Work out the finished part from the listing and answer in its coordinate system (mm). Face numbers are marked on the shaded views. A direction names the side the tool comes from. Coordinates: 2 decimals unless noted, no trailing zeros. Loops run counter-clockwise (first coordinate to the right, second up) from the corner with the lowest first, then second, coordinate; pieces in that order, holes last. Notation, with made-up numbers: (65.5, 50) -> (91.5, 50) arc R31 cw to (91.5, 74) -> close; hole circle Ø8 at (-34.75, -30). An arc over 180 degrees is marked (long way). One line per question, with ' | ' between items.
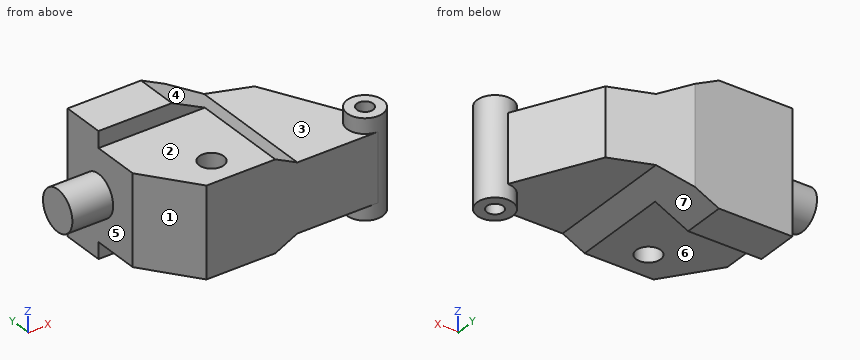
```python
from build123d import *

# Parameters (mm, degrees)
EXTRUDE_1_DEPTH          = 75
SKETCH_2_W               = 185.8
SKETCH_2_H               = 57.3
CUT_EXTRUDE_2_DEPTH      = 120
CUT_EXTRUDE_3_DEPTH      = 400
SKETCH_5_R               = 21.9
EXTRUDE_2_DEPTH          = 60
SKETCH_6_R               = 10
CUT_EXTRUDE_4_DEPTH      = 200
SKETCH_8_R               = 15
CUT_EXTRUDE_5_DEPTH      = 21
CUT_EXTRUDE_5_DEPTH_BACK = 131
SKETCH_9_R               = 25
EXTRUDE_3_DEPTH          = 50


with BuildPart() as part:
    # 草图1 → 凸台-拉伸1 (new body, symmetric)
    with BuildSketch(Plane.XY):
        Polygon((-119.6, 172.501416068), (0, 172.501416068), (86.979350222, 141.023763122), (136.480359145, 43.8), (136.480359145, 0), (-73.719640855, 0), (-119.6, 61.701416068), align=None)
    extrude(amount=EXTRUDE_1_DEPTH, both=True)

    # 草图2 → 切除-拉伸2 (cut)
    with BuildSketch(Plane(origin=(0, 0, 0), x_dir=(1, 0, 0), z_dir=(0, 1, 0))):
        with Locations((-51.7, 83.65)):
            Rectangle(SKETCH_2_W, SKETCH_2_H)
        with Locations((-51.7, -83.65)):
            Rectangle(SKETCH_2_W, SKETCH_2_H)
    extrude(amount=CUT_EXTRUDE_2_DEPTH, mode=Mode.SUBTRACT)

    # 草图3 → 切除-拉伸3 (cut)
    with BuildSketch(Plane(origin=(0, 172.501416068, 0), x_dir=(1, 0, 0), z_dir=(0, 1, 0))):
        Polygon((-64.837283081, 92.42032951), (245.362716919, 92.42032951), (245.362716919, 41.62032951), (37.776604868, 41.62032951), align=None)
        Polygon((37.776604868, -41.62032951), (-64.837283081, -92.42032951), (245.362716919, -92.42032951), (245.362716919, -41.62032951), align=None)
    extrude(amount=-CUT_EXTRUDE_3_DEPTH, mode=Mode.SUBTRACT)

    # 草图5 → 凸台-拉伸2 (add, symmetric)
    with BuildSketch(Plane.XY):
        with Locations((136.480359145, 21.9)):
            Circle(SKETCH_5_R)
    extrude(amount=EXTRUDE_2_DEPTH, both=True)

    # 草图6 → 切除-拉伸4 (cut)
    with BuildSketch(Plane.XY.offset(60)):
        with Locations((136.480359145, 21.9)):
            Circle(SKETCH_6_R)
    extrude(amount=-CUT_EXTRUDE_4_DEPTH, mode=Mode.SUBTRACT)

    # 草图8 → 切除-拉伸5 (cut, two sides)
    with BuildSketch(Plane.XY.offset(55)) as cut_extrude_5_sk:
        with Locations((-42.249773251, 35)):
            Circle(SKETCH_8_R)
    extrude(amount=CUT_EXTRUDE_5_DEPTH, mode=Mode.SUBTRACT)
    extrude(cut_extrude_5_sk.sketch, amount=-CUT_EXTRUDE_5_DEPTH_BACK, mode=Mode.SUBTRACT)

    # 草图9 → 凸台-拉伸3 (add)
    with BuildSketch(Plane.ZY.offset(119.6)):
        with Locations((0, 120)):
            Circle(SKETCH_9_R)
    extrude(amount=EXTRUDE_3_DEPTH)


solid = part.part
```
1) Flat-ended cylindrical pins translate along their axes: pin 1 (8 mm diameter, centred on x = 94, y = 42.5, fed in from +Z); pin 2 (6 mm diameter, centred on x = 2, z = 41.5, fed in from -Y); pin 3 (8 mm diameter, centred on y = 88.5, z = -9.5, fed in from +X); pin 4 (3 mm diameter, centred on x = 27.5, y = 29.5, fed in from -Z). Find the tip coordinate at first contact, or state that the pin passes through.
Check values:
pin 1: stops at z = 41.62 | pin 2: stops at y = 0 | pin 3: stops at x = 115.76 | pin 4: stops at z = -47.45
2) Find section A-A (z = 0). Write down the section's boundary in (x, y), plus the area to 3 significant figures.
Check values:
outline: (-169.6, 95) -> (-119.6, 95) -> (-119.6, 61.7) -> (-73.72, 0) -> (136.48, 0) arc R21.9 ccw to (136.48, 43.8) -> (86.98, 141.02) -> (0, 172.5) -> (-119.6, 172.5) -> (-119.6, 145) -> (-169.6, 145) -> close; hole circle Ø30 at (-42.25, 35); hole circle Ø20 at (136.48, 21.9) | area: 39,700 mm^2
3) Find section B-B (z = -50). Write down the section's boundary in (x, y).
Check values:
outline: (-119.6, 61.7) -> (-73.72, 0) -> (20.85, 0) -> (20.85, 164.96) -> (0, 172.5) -> (-119.6, 172.5) -> close; circle Ø43.8 at (136.48, 21.9); hole circle Ø30 at (-42.25, 35); hole circle Ø20 at (136.48, 21.9)
4) The mould has two halves that part along X. Classify the marked faces 1, 2 and 3: released by +X, released by -X, zero draft, split by the parting line, or undercut.
Check values:
face 1: released by -X | face 2: zero draft | face 3: undercut
5) Find the intervals of material crossed by line 1 along Z through (x, y) = (92, 59); line 2 along Z through (x, y) = (2.5, 16); line 3 along Y through (x, z) = (-52, -56), in increasing order.
Check values:
line 1: z = -41.62 to 41.62 | line 2: z = -55 to 55 | line 3: y = 120 to 172.5
6) For the marked faces 4, 5, 6 and 7, determine the directions among +Z, -Z, +X, -X, +Y, -Y from which every point of the face is accessible in a straight line to the end or side of a thin tool.
Check values:
face 4: +Z, +Y, -Y | face 5: -X | face 6: -Z, -X, -Y | face 7: -Z, +Y, -Y
7) Find section C-C (x = -13). Write down the section's boundary in (y, z), plus the area to 3 significant figures.
Check values:
outline: (0, -55) -> (120, -55) -> (120, -66.76) -> (172.5, -66.76) -> (172.5, 66.76) -> (120, 66.76) -> (120, 55) -> (0, 55) -> close | area: 20,200 mm^2
8) Find section D-D (z = 21.5). Write down the section's boundary in (x, y), plus the area to 3 significant figures.
Check values:
outline: (-169.6, 107.24) -> (-119.6, 107.24) -> (-119.6, 61.7) -> (-73.72, 0) -> (136.48, 0) arc R21.9 ccw to (136.48, 43.8) -> (86.98, 141.02) -> (0, 172.5) -> (-119.6, 172.5) -> (-119.6, 132.76) -> (-169.6, 132.76) -> close; hole circle Ø30 at (-42.25, 35); hole circle Ø20 at (136.48, 21.9) | area: 38,400 mm^2
